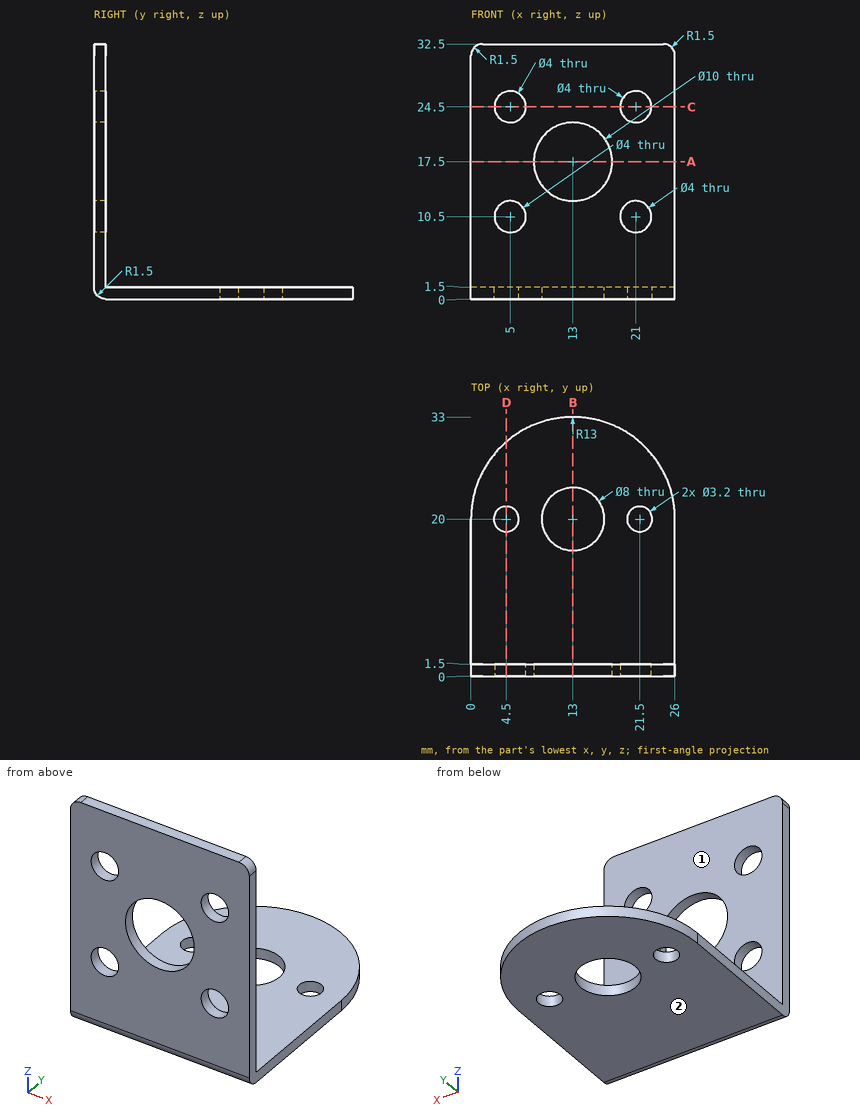
Check sheet for the drawn part. Datum: minimum x, y, z corner. Units: mm. A direction names the side the tool comes from. Round coordinates to 2 decimals unless told otherwise and drop trailing zeros. Write each loop counter-clockwise with the first axis right and the second up, starting at its lowest first coordinate (ties: lowest second). Pieces come first, ordered by that corner, then holes. Notation, with made-up numbers: (-3.5, -18) -> (28.5, -18) arc R25 cw to (28.5, -3) -> close; hole circle Ø2 at (-5, 67). An arc over 180 degrees is marked (long way). Put each result on its own line as item: value.
(1) Go/stop test with flat-tipped pins: pin 1 Ø3 at (x, z) = (13.5, 11) entering from +Y; pin 2 Ø1.5 at (x, y) = (20, 24) entering from +Z. Record where each tip stops, or that it passes through.
Values found:
pin 1: stops at y = 1.5
pin 2: stops at z = 1.5
(2) Sectioned sample at B-B (x = 13). Enter the section's corners in (y, z).
Values found:
outline: (0, 1.5) arc R1.5 ccw to (1.5, 0) -> (16, 0) -> (16, 1.5) -> (1.5, 1.5) -> (1.5, 12.5) -> (0, 12.5) -> close; (0, 22.5) -> (1.5, 22.5) -> (1.5, 32.5) -> (0, 32.5) -> close; (24, 0) -> (33, 0) -> (33, 1.5) -> (24, 1.5) -> close
(3) Sectioned sample at A-A (z = 17.5). Enter the section's corners in (x, y).
Values found:
outline: (0, 0) -> (8, 0) -> (8, 1.5) -> (0, 1.5) -> close; (18, 0) -> (26, 0) -> (26, 1.5) -> (18, 1.5) -> close
(4) Sectioned sample at C-C (z = 24.5). Enter the section's corners in (x, y).
Values found:
outline: (0, 0) -> (3, 0) -> (3, 1.5) -> (0, 1.5) -> close; (7, 0) -> (19, 0) -> (19, 1.5) -> (7, 1.5) -> close; (23, 0) -> (26, 0) -> (26, 1.5) -> (23, 1.5) -> close
(5) Sectioned sample at D-D (x = 4.5). Enter the section's corners in (y, z).
Values found:
outline: (0, 1.5) arc R1.5 ccw to (1.5, 0) -> (18.4, 0) -> (18.4, 1.5) -> (1.5, 1.5) -> (1.5, 8.56) -> (0, 8.56) -> close; (0, 12.44) -> (1.5, 12.44) -> (1.5, 22.56) -> (0, 22.56) -> close; (0, 26.44) -> (1.5, 26.44) -> (1.5, 32.5) -> (0, 32.5) -> close; (21.6, 0) -> (29.84, 0) -> (29.84, 1.5) -> (21.6, 1.5) -> close
(6) Material ranges on line 1 (Z direction, x = 21, y = 0.95); line 2 (X direction, y = 1, z = 10); line 3 (Z direction, x = 15.25, y = 14), recorded low to high.
Values found:
line 1: z = 0.1 to 8.5, 12.5 to 22.5, 26.5 to 32.5
line 2: x = 0 to 3.06, 6.94 to 19.06, 22.94 to 26
line 3: z = 0 to 1.5
(7) Tool access check on the marked faces 1 and 2. Record the directions out of +Z, -Z, +X, -X, +Y, -Y that give a thin tool (end or side, any length) a straight path to the whole face; none if there is none.
Values found:
face 1: +Z, +X, -X, +Y
face 2: -Z, +X, -X, +Y, -Y
